Verification items for the finished model (mm, model axes). A direction names the side the tool comes from. Give positions to 0.01 mm unless a question says otherwise; leave off trailing zeros. Loops run counter-clockwise (first coordinate to the right, second up) from the corner with the lowest first, then second, coordinate; pieces in that order, holes last. Notation, with made-up numbers: M 5.25,69.5 L 10.25,69.5 A21 ccw 10.25,106.5 Z; hole C 40,38 d4. An arc over 180 degrees is marked long. Use a Markdown table: item, result.
from build123d import *

# Parameters (mm, degrees)
BOSS_EXTRUDE1_DEPTH = 12.7
CUT_EXTRUDE1_DEPTH  = 9.525
CUT_EXTRUDE2_DEPTH  = 6.35
CUT_EXTRUDE3_DEPTH  = 9.525
SKETCH5_R           = 1.5
CUT_EXTRUDE4_DEPTH  = 3.175


with BuildPart() as part:
    # Sketch1 → Boss-Extrude1 (new body)
    with BuildSketch(Plane.XY):
        with BuildLine():
            Line((48.378329117, 83.793724016), (90, 155.884572681))
            ThreePointArc((90, 155.884572681), (46.587428118, 173.866648732), (0, 180))
            Line((0, 180), (0, 96.756658234))
            ThreePointArc((0, 96.756658234), (25.042465891, 93.459755054), (48.378329117, 83.793724016))
        make_face()
    extrude(amount=BOSS_EXTRUDE1_DEPTH)

    # Sketch2 → Cut-Extrude1 (cut)
    with BuildSketch(Plane.XY.offset(12.7)):
        with BuildLine():
            Line((0, 100), (0, 167.5))
            ThreePointArc((0, 167.5), (43.352190055, 161.792575903), (83.75, 145.059255134))
            Line((83.75, 145.059255134), (50, 86.602540378))
            ThreePointArc((50, 86.602540378), (25.88190451, 96.592582629), (0, 100))
        make_face()
    extrude(amount=-CUT_EXTRUDE1_DEPTH, mode=Mode.SUBTRACT)

    # Sketch3 → Cut-Extrude2 (cut)
    with BuildSketch(Plane.XY.offset(12.7)):
        with BuildLine():
            Line((48.378329117, 83.793724016), (50, 86.602540378))
            ThreePointArc((50, 86.602540378), (25.88190451, 96.592582629), (0, 100))
            Line((0, 100), (0, 96.756658234))
            ThreePointArc((0, 96.756658234), (25.042465891, 93.459755054), (48.378329117, 83.793724016))
        make_face()
    extrude(amount=-CUT_EXTRUDE2_DEPTH, mode=Mode.SUBTRACT)

    # Sketch4 → Cut-Extrude3 (cut)
    with BuildSketch(Plane(origin=(0, 0, 0), x_dir=(-1, 0, 0), z_dir=(0, 0, -1))):
        with BuildLine():
            Line((0, 169.5), (0, 180))
            ThreePointArc((0, 180), (-46.587428118, 173.866648732), (-90, 155.884572681))
            Line((-90, 155.884572681), (-84.75, 146.791305941))
            ThreePointArc((-84.75, 146.791305941), (-43.869828145, 163.724427556), (0, 169.5))
        make_face()
    extrude(amount=-CUT_EXTRUDE3_DEPTH, mode=Mode.SUBTRACT)

    # Sketch5 → Cut-Extrude4 (cut)
    with BuildSketch(Plane(origin=(0, 0, 9.525), x_dir=(-1, 0, 0), z_dir=(0, 0, -1))):
        with Locations((-22.80945209, 173.254989525)):
            Circle(SKETCH5_R)
        with Locations(Location((-66.873929806, 161.447948306, 0), (0, 0, 180))):
            Circle(SKETCH5_R)
    extrude(amount=-CUT_EXTRUDE4_DEPTH, mode=Mode.SUBTRACT)


solid = part.part
(1) Set-up check for faces 5 (the flat face through (25, 94, 6.35)), 6 (the cylindrical face through (44.47, 163.563, 4.696)), 7 (the flat face through (32, 127, 0)), 8 (the flat face through (69.09, 119.67, 2.56)), 9 (the cylindrical face through (42.76, 161.95, 8)): record each of +Z, -Z, +X, -X, +Y, -Y from which the full face is reachable in a straight line by a thin tool's end or side.
Results below:
| item | result |
|---|---|
| face 5 | +Z, +X, -X, -Y |
| face 6 | -Z, +X, +Y |
| face 7 | -Z, +X, -X, +Y, -Y |
| face 8 | +Z, -Z, +X, -Y |
| face 9 | +Z, -X |
(2) Cross-section at D-D on y = 98. Record the cut outline in (x, z) (3 decimals), then the cut area to 3 significant figures.
Results below:
| item | result |
|---|---|
| outline | M 0,0 L 56.58,0 L 56.58,3.175 L 19.9,3.175 L 19.9,6.35 L 0,6.35 Z |
| area | 243 mm^2 |
(3) Cross-section at A-A on z = 4.25. Record the cut outline in (x, y), then the cut area to 3 significant figures.
Results below:
| item | result |
|---|---|
| outline | M 0,96.76 A96.76 cw 48.38,83.79 L 50,86.6 A100 ccw 0,100 Z; M 0,167.5 A167.5 cw 83.75,145.06 L 84.75,146.79 A169.5 ccw 0,169.5 Z |
| area | 344 mm^2 |
(4) Cross-section at B-B on x = 78. Record the cut outline in (y, z) (3 decimals), then the cut area to 3 significant figures.
Results below:
| item | result |
|---|---|
| outline | M 135.1,0 L 150.487,0 L 150.487,9.525 L 162.222,9.525 L 162.222,12.7 L 148.23,12.7 L 148.23,3.175 L 135.1,3.175 Z |
| area | 108 mm^2 |
(5) Material ranges on line 1 (Z direction, x = 70, y = 135) (3 decimals); line 2 (Z direction, x = 41.5, y = 88.5); line 3 (Y direction, x = 46, z = 4.75), recorded low to high.
Results below:
| item | result |
|---|---|
| line 1 | 0 to 3.175 |
| line 2 | 0 to 6.35 |
| line 3 | 85.12 to 88.79, 161.06 to 163.14 |
(6) Draft check along X on faces 1 (the flat face through (0, 139, 3)), 2 (the cylindrical face through (23.13, 171.79, 11.09)), 3 (the cylindrical face through (66.5, 162.9, 11.1)), 4 (the cylindrical face through (26.236, 96.497, 4.785)). Enter one of: +X half, -X half, draft (parallel to the pull), parting line (faces both ways), or undercut.
Results below:
| item | result |
|---|---|
| face 1 | -X half |
| face 2 | undercut |
| face 3 | undercut |
| face 4 | +X half |
(7) Cross-section at C-C on z = 10.75. Record the cut outline in (x, y), then the cut area to 3 significant figures.
Results below:
| item | result |
|---|---|
| outline | M 0,167.5 A167.5 cw 83.75,145.06 L 90,155.88 A180 ccw 0,180 Z; hole C 22.81,173.25 d3; hole C 66.87,161.45 d3 |
| area | 1,120 mm^2 |
(8) Gauge pin test, flat ends, axial feed: P1, Ø5, axis at x = 32, z = 9, coming from the -Y side; P2, Ø2.5, axis at x = 22.81, y = 173.25, coming from the -Z side; P3, Ø24.5, axis at x = 41.5, y = 146.5, coming from the +Z side (3 decimals); P4, Ø4, axis at x = 76.5, z = 11, coming from the +Y side. Record the tip position at first contact, or that the pin passes through.
Results below:
| item | result |
|---|---|
| P1 | y = 163.91 |
| P2 | through |
| P3 | z = 3.175 |
| P4 | y = 163.86 |
